```python
from build123d import *

# Parameters (mm, degrees)
BOX031_W                 = 46
BOX031_H                 = 15
BOX031_DEPTH             = 16
BOX029_W                 = 78
BOX029_H                 = 15
BOX029_DEPTH             = 6
BOX023_W                 = 220
BOX023_H                 = 2.5
BOX023_DEPTH             = 3
EXTRUDE011_DEPTH         = 10
BOX024_W                 = 220
BOX024_H                 = 113
BOX024_DEPTH             = 8
BOX026_W                 = 32
BOX026_H                 = 6
BOX026_DEPTH             = 6
PRISM004_DEPTH           = 6
PRISM004_PLACEMENT_ANGLE = 30
PRISM005_DEPTH           = 6
PRISM005_PLACEMENT_ANGLE = 30
EXTRUDE012_DEPTH         = 39
EXTRUDE009_DEPTH         = 39
EXTRUDE008_DEPTH         = 39
BOX009_W                 = 12.5
BOX009_H                 = 7.5
BOX009_DEPTH             = 22
BOX010_W                 = 12.5
BOX010_H                 = 7.5
BOX010_DEPTH             = 22
CYLINDER_R               = 1.7
CYLINDER_DEPTH           = 30
BOX007_W                 = 15
BOX007_H                 = 70
BOX007_DEPTH             = 6
BOX006_W                 = 40
BOX006_H                 = 51
BOX006_DEPTH             = 6
EXTRUDE010_DEPTH         = 39
BOX021_W                 = 12.5
BOX021_H                 = 7.5
BOX021_DEPTH             = 22
BOX027_W                 = 12.5
BOX027_H                 = 7.5
BOX027_DEPTH             = 22
CYLINDER002_R            = 1.7
CYLINDER002_DEPTH        = 30
BOX025_W                 = 15
BOX025_H                 = 70
BOX025_DEPTH             = 6
BOX022_W                 = 40
BOX022_H                 = 51
BOX022_DEPTH             = 6
BOX005_W                 = 20
BOX005_H                 = 6
BOX005_DEPTH             = 30
BOX004_W                 = 40
BOX004_H                 = 6
BOX004_DEPTH             = 44.5


with BuildPart() as cube030:
    # Box031 → Box031 (new body)
    with BuildSketch(Plane(origin=(-22, 15, 0), x_dir=(1, 0, 0), z_dir=(0, 0, 1))):
        with Locations((23, 7.5)):
            Rectangle(BOX031_W, BOX031_H)
    extrude(amount=BOX031_DEPTH)


with BuildPart() as cube028:
    # Box029 → Box029 (new body)
    with BuildSketch(Plane(origin=(-39, 0, 0), x_dir=(1, 0, 0), z_dir=(0, 0, 1))):
        with Locations((39, 7.5)):
            Rectangle(BOX029_W, BOX029_H)
    extrude(amount=BOX029_DEPTH)


with BuildPart() as cube022:
    # Box023 → Box023 (new body)
    with BuildSketch(Plane(origin=(-110, 2, 0), x_dir=(1, 0, 0), z_dir=(0, 0, 1))):
        with Locations((110, 1.25)):
            Rectangle(BOX023_W, BOX023_H)
    extrude(amount=BOX023_DEPTH)


with BuildPart() as extrude011:
    # Sketch009 → Extrude011 (new body)
    with BuildSketch(Plane.XY):
        Polygon((-95, 0), (95, 0), (85, 61), (-85, 61), align=None)
    extrude(amount=EXTRUDE011_DEPTH)


with BuildPart() as obj1:
    # Box024 → Box024 (new body)
    with BuildSketch(Plane(origin=(-110, -15, 0), x_dir=(1, 0, 0), z_dir=(0, 0, 1))):
        with Locations((110, 56.5)):
            Rectangle(BOX024_W, BOX024_H)
    extrude(amount=BOX024_DEPTH)

    # Cut004020: cut Extrude011
    add(extrude011.part, mode=Mode.SUBTRACT)


with BuildPart() as cube025:
    # Box026 → Box026 (new body)
    with BuildSketch(Plane(origin=(-16, 55, 0), x_dir=(1, 0, 0), z_dir=(0, 0, 1))):
        with Locations((16, 3)):
            Rectangle(BOX026_W, BOX026_H)
    extrude(amount=BOX026_DEPTH)


with BuildPart() as prism004:
    # Prism004 → Prism004 (new body)
    with BuildSketch(Plane.XY):
        Polygon((45, 0), (-22.5, 38.971143), (-22.5, -38.971143), align=None)
    extrude(amount=PRISM004_DEPTH)


with BuildPart() as prism004_1:
    # Prism004 placement: moved
    add(prism004.part.moved(Location((0, 23, 0))).rotate(Axis((0, 23, 0), (0, 0, -1)), PRISM004_PLACEMENT_ANGLE))


with BuildPart() as obj2:
    # Prism005 → Prism005 (new body)
    with BuildSketch(Plane.XY):
        Polygon((60, 0), (-30, 51.961524), (-30, -51.961524), align=None)
    extrude(amount=PRISM005_DEPTH)


with BuildPart() as obj2_1:
    # Prism005 placement: moved
    add(obj2.part.moved(Location((0, 23, 0))).rotate(Axis((0, 23, 0), (0, 0, -1)), PRISM005_PLACEMENT_ANGLE))

    # Cut004019: cut Prism004
    add(prism004_1.part, mode=Mode.SUBTRACT)


with BuildPart() as obj2_2:
    # Cut004019 placement: moved
    add(obj2_1.part.moved(Location((0, 7, 0))))

    # Fusion004005: union Cube025
    add(cube025.part)

    # Cut004015: cut obj1
    add(obj1.part, mode=Mode.SUBTRACT)

    # Cut004016: cut Cube022
    add(cube022.part, mode=Mode.SUBTRACT)


with BuildPart() as extrude012:
    # Sketch010 (on Face21 of Fusion004006) → Extrude012 (new body)
    with BuildSketch(Plane(origin=(-20, 0, 0), x_dir=(0, -1, 0), z_dir=(-1, 0, 0))):
        Polygon((-7.5, 0), (-7.5, 25), (-21.933757, 0), align=None)
    extrude(amount=-EXTRUDE012_DEPTH)


with BuildPart() as extrude012_1:
    # Extrude012 placement: moved
    add(extrude012.part.moved(Location((27.5, 0, 0))))


with BuildPart() as extrude009:
    # Sketch007 (on Face17 of Fusion004002) → Extrude009 (new body)
    with BuildSketch(Plane(origin=(-20, 0, 0), x_dir=(0, -1, 0), z_dir=(-1, 0, 0))):
        Polygon((0, 0), (0, 19), (45, 19), align=None)
    extrude(amount=EXTRUDE009_DEPTH)


with BuildPart() as extrude009_1:
    # Extrude009 placement: moved
    add(extrude009.part.moved(Location((66.5, 0, 0))))


with BuildPart() as extrude008:
    # Sketch007 (on Face17 of Fusion004002) → Extrude008 (new body)
    with BuildSketch(Plane(origin=(-20, 0, 0), x_dir=(0, -1, 0), z_dir=(-1, 0, 0))):
        Polygon((0, 0), (0, 19), (45, 19), align=None)
    extrude(amount=-EXTRUDE008_DEPTH)


with BuildPart() as extrude008_1:
    # Extrude008 placement: moved
    add(extrude008.part.moved(Location((-26.5, 0, 0))))


with BuildPart() as cube008:
    # Box009 → Box009 (new body)
    with BuildSketch(Plane(origin=(7.5, 0, 3), x_dir=(1, 0, 0), z_dir=(0, 0, 1))):
        with Locations((6.25, 3.75)):
            Rectangle(BOX009_W, BOX009_H)
    extrude(amount=BOX009_DEPTH)


with BuildPart() as cube009:
    # Box010 → Box010 (new body)
    with BuildSketch(Plane(origin=(-20, 0, 3), x_dir=(1, 0, 0), z_dir=(0, 0, 1))):
        with Locations((6.25, 3.75)):
            Rectangle(BOX010_W, BOX010_H)
    extrude(amount=BOX010_DEPTH)


with BuildPart() as cylinder:
    # Cylinder → Cylinder (new body)
    with BuildSketch(Plane(origin=(0, 7, 0), x_dir=(1, 0, 0), z_dir=(0, 0, 1))):
        Circle(CYLINDER_R)
    extrude(amount=CYLINDER_DEPTH)


with BuildPart() as cube007:
    # Box007 → Box007 (new body)
    with BuildSketch(Plane(origin=(12.5, 22, 20), x_dir=(1, 0, 0), z_dir=(0, 0, 1))):
        with Locations((7.5, 35)):
            Rectangle(BOX007_W, BOX007_H)
    extrude(amount=BOX007_DEPTH)


with BuildPart() as fusion004002:
    # Box006 → Box006 (new body)
    with BuildSketch(Plane.XY.offset(20)):
        with Locations((20, 25.5)):
            Rectangle(BOX006_W, BOX006_H)
    extrude(amount=BOX006_DEPTH)

    # Cut004005: cut Cube007
    add(cube007.part, mode=Mode.SUBTRACT)


with BuildPart() as fusion004002_1:
    # Cut004005 placement: moved
    add(fusion004002.part.moved(Location((-20, 0, -1))))

    # Cut004006: cut Cylinder
    add(cylinder.part, mode=Mode.SUBTRACT)


with BuildPart() as fusion004002_2:
    # Cut004006 placement: moved
    add(fusion004002_1.part.moved(Location((0, -45, 0))))

    # Fusion004002: union Cube008, Cube009
    add(cube008.part)
    add(cube009.part)


with BuildPart() as fusion004007:
    # Sketch008 (on Face21 of Fusion004002) → Extrude010 (new body)
    with BuildSketch(Plane(origin=(-20, 0, 0), x_dir=(0, -1, 0), z_dir=(-1, 0, 0))):
        Polygon((-7.5, 0), (-7.5, 25), (-21.933757, 0), align=None)
    extrude(amount=-EXTRUDE010_DEPTH)


with BuildPart() as fusion004007_1:
    # Extrude010 placement: moved
    add(fusion004007.part.moved(Location((-26.5, 0, 0))))

    # Fusion004007: union Extrude012, Extrude009, Extrude008, Fusion004002
    add(extrude012_1.part)
    add(extrude009_1.part)
    add(extrude008_1.part)
    add(fusion004002_2.part)


with BuildPart() as cube020:
    # Box021 → Box021 (new body)
    with BuildSketch(Plane(origin=(7.5, 0, 3), x_dir=(1, 0, 0), z_dir=(0, 0, 1))):
        with Locations((6.25, 3.75)):
            Rectangle(BOX021_W, BOX021_H)
    extrude(amount=BOX021_DEPTH)


with BuildPart() as cube026:
    # Box027 → Box027 (new body)
    with BuildSketch(Plane(origin=(-20, 0, 3), x_dir=(1, 0, 0), z_dir=(0, 0, 1))):
        with Locations((6.25, 3.75)):
            Rectangle(BOX027_W, BOX027_H)
    extrude(amount=BOX027_DEPTH)


with BuildPart() as cylinder002:
    # Cylinder002 → Cylinder002 (new body)
    with BuildSketch(Plane(origin=(0, 7, 0), x_dir=(1, 0, 0), z_dir=(0, 0, 1))):
        Circle(CYLINDER002_R)
    extrude(amount=CYLINDER002_DEPTH)


with BuildPart() as cube024:
    # Box025 → Box025 (new body)
    with BuildSketch(Plane(origin=(12.5, 22, 20), x_dir=(1, 0, 0), z_dir=(0, 0, 1))):
        with Locations((7.5, 35)):
            Rectangle(BOX025_W, BOX025_H)
    extrude(amount=BOX025_DEPTH)


with BuildPart() as parte_frontal:
    # Box022 → Box022 (new body)
    with BuildSketch(Plane.XY.offset(20)):
        with Locations((20, 25.5)):
            Rectangle(BOX022_W, BOX022_H)
    extrude(amount=BOX022_DEPTH)

    # Cut004017: cut Cube024
    add(cube024.part, mode=Mode.SUBTRACT)


with BuildPart() as parte_frontal_1:
    # Cut004017 placement: moved
    add(parte_frontal.part.moved(Location((-20, 0, -1))))

    # Cut004018: cut Cylinder002
    add(cylinder002.part, mode=Mode.SUBTRACT)


with BuildPart() as parte_frontal_2:
    # Cut004018 placement: moved
    add(parte_frontal_1.part.moved(Location((0, -45, 0))))

    # Fusion004006: union Cube020, Cube026
    add(cube020.part)
    add(cube026.part)

    # Fusion004008: union Fusion004007
    add(fusion004007_1.part)


with BuildPart() as cube005:
    # Box005 → Box005 (new body)
    with BuildSketch(Plane(origin=(-10, 55, 6), x_dir=(1, 0, 0), z_dir=(0, 0, 1))):
        with Locations((10, 3)):
            Rectangle(BOX005_W, BOX005_H)
    extrude(amount=BOX005_DEPTH)


with BuildPart() as cut004022:
    # Box004 → Box004 (new body)
    with BuildSketch(Plane(origin=(-20, 55, 0), x_dir=(1, 0, 0), z_dir=(0, 0, 1))):
        with Locations((20, 3)):
            Rectangle(BOX004_W, BOX004_H)
    extrude(amount=BOX004_DEPTH)

    # Cut004004: cut Cube005
    add(cube005.part, mode=Mode.SUBTRACT)

    # Fusion004009: union obj2, parte_frontal
    add(obj2_2.part)
    add(parte_frontal_2.part)

    # Fusion004009002: union Cube028
    add(cube028.part)

    # Cut004022: cut Cube030
    add(cube030.part, mode=Mode.SUBTRACT)


solid = cut004022.part
```
Verification items for the finished model (mm, model axes). A direction names the side the tool comes from. Round coordinates to 2 decimals unless told otherwise and drop trailing zeros. Order: outer loops, then holes, each group sorted by start corner. A loop starts at its lowest first (then second) coordinate and runs counter-clockwise, first axis right, second up. Notation, with made-up numbers: (80.5, -5.5) -> (133.5, -5.5) arc R12 cw to (133.5, 12.5) -> close; hole circle Ø5 at (-36.75, -11). An arc over 180 degrees is marked (long way). Put each result on its own line as item: value. Start each with the question number.
(1) Draft check along X on faces 1 (the face through (39, 3, 1)), 2 (the face through (0, -34, 19)), 3 (the face through (45, 3, 3)). Enter one of: +X half, -X half, draft (parallel to the pull), parting line (faces both ways), or undercut.
(2) Tool access check on faces 4 (the face through (46.5, 12, 7)), 5 (the face through (-45, 2, 1)), 6 (the face through (44, 4.5, 1)). Record the directions out of +Z, -Z, +X, -X, +Y, -Y that give a thin tool (end or side, any length) a straight path to the whole face; none if there is none.
(3) Depth check by flat-ended pin: pin 1 Ø6.5 at (x, z) = (34, 10) entering from +Y; pin 2 Ø12 at (x, y) = (-27, 15.5) entering from +Z; pin 3 Ø21 at (x, y) = (-27, -28.5) entering from +Z. Enter the tip coordinate at first touch or a pass-through.
(4) Section check D-D (z = 15.5). Enter the section's corners in (x, y), then the cut area to 3 significant figures.
(5) Material ranges on line 1 along Y through (x, z) = (0, 22.05); line 2 along X through (y, z) = (-38, 22); line 3 along Z through (x, y) = (7, 3), recorded low to high.
(6) Section check A-A (x = -44.5). Enter the section's corners in (y, z).
(7) Section check B-B (y = -16.5). Enter the section's corners in (x, z).
(8) Section check C-C (x = -13.5). Enter the section's corners in (y, z), then the cut area to 3 significant figures.
Completed:
1. face 1: +X half
1. face 2: undercut
1. face 3: draft
2. face 4: +Z, +X, +Y
2. face 5: -Z, -X
2. face 6: -Z, +X
3. pin 1: stops at y = 18.04
3. pin 2: stops at z = 21.54
3. pin 3: stops at z = 25
4. outline: (-46.5, -36.71) -> (-7.5, -36.71) -> (-7.5, 12.98) -> (-46.5, 12.98) -> (-46.5, 7.5) -> (-20, 7.5) -> (-20, 0) -> (-46.5, 0) -> close; (-20, 55) -> (-10, 55) -> (-10, 61) -> (-20, 61) -> close; (7.5, -36.71) -> (46.5, -36.71) -> (46.5, 0) -> (20, 0) -> (20, 7.5) -> (46.5, 7.5) -> (46.5, 12.98) -> (7.5, 12.98) -> close; (10, 55) -> (20, 55) -> (20, 61) -> (10, 61) -> close
4. area: 3,600 mm2
5. line 1: y = -45 to -39.7, -36.3 to -23
5. line 2: x = -20 to -1.7, 1.7 to 20
5. line 3: z = 0 to 6
6. outline: (-45, 19) -> (0, 0) -> (2, 0) -> (2, 3) -> (4.5, 3) -> (4.5, 0) -> (21.93, 0) -> (7.5, 25) -> (7.5, 6) -> (0, 6) -> (0, 19) -> close
7. outline: (-46.5, 6.97) -> (-7.5, 6.97) -> (-7.5, 25) -> (-20, 25) -> (-20, 19) -> (-46.5, 19) -> close; (7.5, 6.97) -> (46.5, 6.97) -> (46.5, 19) -> (20, 19) -> (20, 25) -> (7.5, 25) -> close
8. outline: (-45, 19) -> (0, 0) -> (15, 0) -> (15, 12.01) -> (7.5, 25) -> (-45, 25) -> close; (51.62, 0) -> (61, 0) -> (61, 44.5) -> (55, 44.5) -> (55, 6) -> (51.62, 6) -> close
8. area: 1,310 mm2
